```python
from build123d import *

# Parameters (mm, degrees)
SKETCH_1_R      = 10
EXTRUDE_1_DEPTH = 288.75
M10X1_5_1_D     = 8.5
M10X1_5_1_DEPTH = 24.5
M10X1_5_1_TIP   = 2.553657631
CHAMFER_1_SIZE  = 1


with BuildPart() as part:
    # 草图1 → 凸台-拉伸1 (new, symmetric)
    with BuildSketch(Plane(origin=(0, 0, 0), x_dir=(0, 0, -1), z_dir=(1, 0, 0))):
        Circle(SKETCH_1_R)
    extrude(amount=EXTRUDE_1_DEPTH, both=True)

    # M10x1.5 螺纹孔1
    with Locations(Plane(origin=(288.75, 0, 0), x_dir=(0, 0, -1), z_dir=(1, 0, 0))):
        with Locations((0, 0)):
            Hole(M10X1_5_1_D / 2, depth=M10X1_5_1_DEPTH)
            with Locations((0, 0, -(M10X1_5_1_DEPTH + M10X1_5_1_TIP / 2))):  # 118° drill point
                Cone(0, M10X1_5_1_D / 2, M10X1_5_1_TIP, mode=Mode.SUBTRACT)

    # 倒角1
    chamfer_1_edges = [part.edges().sort_by_distance(p)[0] for p in [
        (-288.75, 0, 10),
        (288.75, 0, 10),
    ]]
    chamfer(chamfer_1_edges, length=CHAMFER_1_SIZE)


solid = part.part
```
Check sheet for the modelled part. Datum: model origin and axes. Units: mm. Give positions to 0.01 mm unless a question says otherwise; leave off trailing zeros. Write each loop counter-clockwise with the first axis right and the second up, starting at its lowest first coordinate (ties: lowest second). Pieces come first, ordered by that corner, then holes.
Item 1: Cross-section at A-A (x = -212.5). Enter the section's corners in (y, z), and give its area (3 significant figures).
Item 2: Scan lines: L1, parallel to Y at x = 274.25, z = 0; L2, parallel to Y at x = -56, z = 1.25; L3, parallel to Y at x = 122.5, z = 3.5. Record each from-to range of solid material in increasing order.
Item 3: Gauge pin test, flat ends, axial feed: pin 1 (10 mm diameter, centred on x = -88, y = 5.5, fed in from +Z); pin 2 (3 mm diameter, centred on x = 20, y = -4.5, fed in from -Z); pin 3 (8 mm diameter, centred on x = -5, z = -5, fed in from -Y). Record the tip position at first contact, or that the pin passes through.
Report:
1. outline: circle Ø20 at (0, 0)
1. area: 314 mm2
2. L1: y = -10 to -4.25, 4.25 to 10
2. L2: y = -9.92 to 9.92
2. L3: y = -9.37 to 9.37
3. pin 1: stops at z = 9.99
3. pin 2: stops at z = -9.54
3. pin 3: stops at y = -9.95
